Verification items for this drawing (mm, ordinates from the low corner). Round coordinates to 2 decimals unless told otherwise and drop trailing zeros. Write each loop counter-clockwise with the first axis right and the second up, starting at its lowest first coordinate (ties: lowest second). Pieces come first, ordered by that corner, then holes. Notation, with made-up numbers: (-4.5, 33.25) -> (2.5, 33.25) arc R19 cw to (2.5, 46.25) -> close; hole circle Ø6 at (-33.75, 54.25). An arc over 180 degrees is marked (long way). One line per item, written item: value.
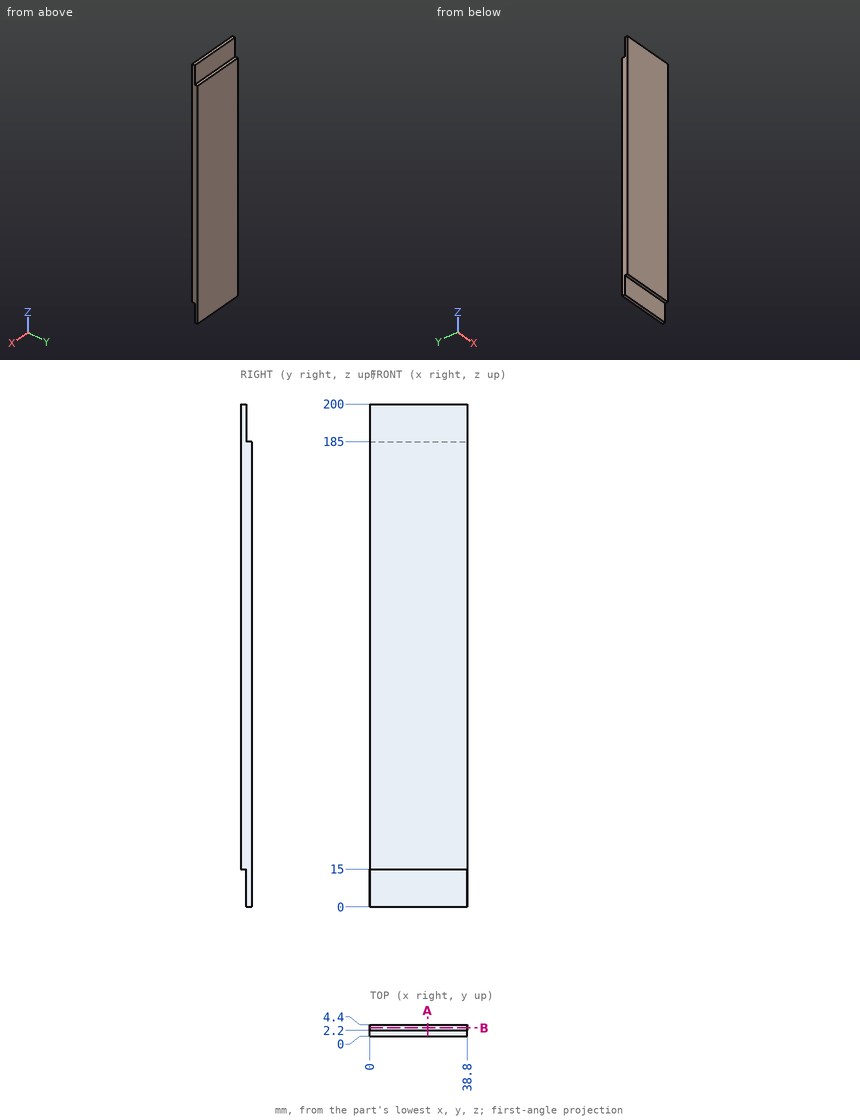
Item 1: Depth check by flat-ended pin: pin 1 (1.1 mm diameter, centred on x = 10.5, y = 0.5, fed in from -Z); pin 2 (7.5 mm diameter, centred on x = 19.5, z = 5.5, fed in from -Y); pin 3 (7.5 mm diameter, centred on x = 20.5, z = 193.5, fed in from +Y). Enter the tip coordinate at first touch or a pass-through.
Result set:
pin 1: z = 15
pin 2: y = 2.2
pin 3: y = 2.2
Item 2: Material ranges on line 1 along Z through (x, y) = (27, 2.5); line 2 along Z through (x, y) = (14, 1.4); line 3 along Y through (x, z) = (36.5, 188.5), recorded low to high.
Result set:
line 1: 0 to 185
line 2: 15 to 200
line 3: 0 to 2.2
Item 3: Sectioned sample at B-B (y = 3.25). Enter the section's corners in (x, z).
Result set:
outline: (0, 0) -> (38.8, 0) -> (38.8, 185) -> (0, 185) -> close
Item 4: Sectioned sample at A-A (x = 23). Enter the section's corners in (y, z).
Result set:
outline: (0, 15) -> (2.2, 15) -> (2.2, 0) -> (4.4, 0) -> (4.4, 185) -> (2.2, 185) -> (2.2, 200) -> (0, 200) -> close
